Source: CAD feature listing. Evaluate the final solid. Frame: model axes, mm. Face numbers are marked on the shaded views. A direction names the side the tool comes from. Give positions to 0.01 mm unless a question says otherwise; leave off trailing zeros. Write each loop counter-clockwise with the first axis right and the second up, starting at its lowest first coordinate (ties: lowest second). Pieces come first, ordered by that corner, then holes. Notation, with made-up numbers: (-22.5, 13.25) -> (8.5, 13.25) arc R12 ccw to (8.5, 18.25) -> close; hole circle Ø1 at (4, 63). An arc over 180 degrees is marked (long way). Use a Markdown table: item, result. Add a question column.
```python
from build123d import *

# Parameters (mm, degrees)
SFAZOWANIE1_SIZE           = 1
SFAZOWANIE2_SIZE           = 0.5
WYTNIJ_WYCI_GNI_CIE1_START = -25
WYTNIJ_WYCI_GNI_CIE1_DEPTH = 25


with BuildPart() as part:
    # Szkic1 → Obrót1 (revolve)
    with BuildSketch(Plane.XY, mode=Mode.PRIVATE) as obr_t1_sk:
        Polygon((0, 0), (0, 5), (0.6, 5), (0.6, 4.6), (1.7, 4.6), (1.7, 5), (10.7, 5), (10.7, 5.5), (22.7, 5.5), (22.7, 7.5), (47.7, 7.5), (47.7, 10.2), (67.7, 10.2), (67.7, 9.5), (101.7, 9.5), (101.7, 10.2), (121.7, 10.2), (121.7, 12.25), (124.7, 12.25), (124.7, 5), (133.7, 5), (133.7, 4.6), (134.8, 4.6), (134.8, 5), (135.4, 5), (135.4, 0), align=None)
    revolve(obr_t1_sk.sketch.rotate(Axis((-10.674656103, 0, 0), (1, 0, 0)), 90), axis=Axis((-10.674656103, 0, 0), (1, 0, 0)))

    # Sfazowanie1
    # the kernel refuses this chamfer: 1 mm, written as the material it takes off along each edge
    with BuildSketch(Plane(origin=(101.7, 0, 0), x_dir=(0, 0, 1), z_dir=(0, 1, 0))) as sfazowanie1_piece_1_section:
        Polygon((10.2 - SFAZOWANIE1_SIZE, 0), (10.2, SFAZOWANIE1_SIZE), (10.2, 0), align=None)
    sfazowanie1_piece_1 = revolve(axis=Axis((101.7, 0, 0), (1, 0, 0)), mode=Mode.PRIVATE)
    sfazowanie1_piece_1 = sfazowanie1_piece_1 - Plane(origin=(102.341981052, 0, 0), x_dir=(0, 0, 1), z_dir=(1, 0, 0)) * Cylinder(9.5, 41, mode=Mode.PRIVATE)
    add(sfazowanie1_piece_1, mode=Mode.SUBTRACT)
    with BuildSketch(Plane(origin=(67.7, 0, 0), x_dir=(0, 0, 1), z_dir=(0, 1, 0))) as sfazowanie1_piece_2_section:
        Polygon((10.2, -SFAZOWANIE1_SIZE), (10.2 - SFAZOWANIE1_SIZE, 0), (10.2, 0), align=None)
    sfazowanie1_piece_2 = revolve(axis=Axis((67.7, 0, 0), (1, 0, 0)), mode=Mode.PRIVATE)
    sfazowanie1_piece_2 = sfazowanie1_piece_2 - Plane(origin=(67.058018948, 0, 0), x_dir=(0, 0, 1), z_dir=(1, 0, 0)) * Cylinder(9.5, 41, mode=Mode.PRIVATE)
    add(sfazowanie1_piece_2, mode=Mode.SUBTRACT)
    with BuildSketch(Plane(origin=(124.7, 0, 0), x_dir=(0, 0, 1), z_dir=(0, 1, 0))) as sfazowanie1_piece_3:
        Polygon((12.25, -SFAZOWANIE1_SIZE), (12.25 - SFAZOWANIE1_SIZE, 0), (12.25, 0), align=None)
    revolve(axis=Axis((124.7, 0, 0), (1, 0, 0)), mode=Mode.SUBTRACT)
    with BuildSketch(Plane(origin=(47.7, 0, 0), x_dir=(0, 0, 1), z_dir=(0, 1, 0))) as sfazowanie1_piece_4:
        Polygon((10.2 - SFAZOWANIE1_SIZE, 0), (10.2, SFAZOWANIE1_SIZE), (10.2, 0), align=None)
    revolve(axis=Axis((47.7, 0, 0), (1, 0, 0)), mode=Mode.SUBTRACT)

    # Sfazowanie2
    sfazowanie2_edges = [part.edges().sort_by_distance(p)[0] for p in [
        (135.4, 0, -5),
        (0, 0, -5),
    ]]
    chamfer(sfazowanie2_edges, length=SFAZOWANIE2_SIZE)

    # Szkic2 → Wytnij-wyciągnięcie1 (cut)
    with BuildSketch(Plane.ZY.offset(-22.7).offset(WYTNIJ_WYCI_GNI_CIE1_START)):
        with BuildLine():
            Line((4.5, -6), (-4.5, -6))
            ThreePointArc((-4.5, -6), (0, -7.5), (4.5, -6))
        make_face()
    extrude(amount=WYTNIJ_WYCI_GNI_CIE1_DEPTH, mode=Mode.SUBTRACT)


solid = part.part
```
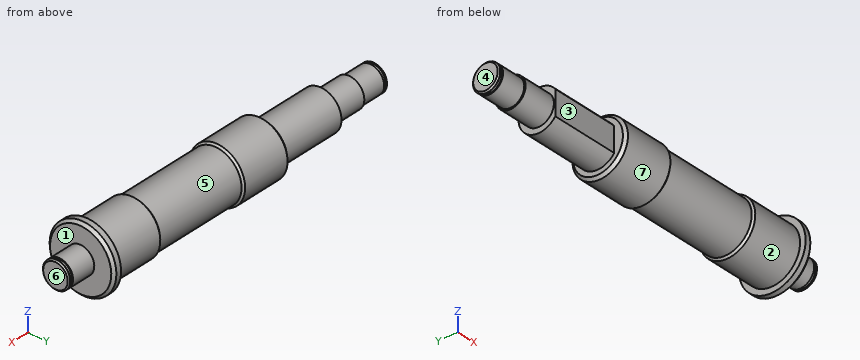
(1) Mould query, pull axis X, two halves, no side actions, for the marked faces 4, 5, 6 and 7. Classes: +X half, -X half, draft (parallel to the pull), parting line (faces both ways), or undercut.
(2) Cut plane B-B on x = 43. Return the cut outline in (y, z), then the cut area to 3 significant figures.
(3) Cut plane A-A on x = 63.5. Return the cut outline in (y, z).
(4) Material intervals for L1, parallel to X at y = -3.75, z = -3; L2, parallel to X at y = 10.5, z = -0.75; L3, parallel to Z at x = 116, y = -0.75, sorted ascending.
(5) Access query for the marked faces 1, 2 and 3. Directions: +Z, -Z, +X, -X, +Y, -Y. A direction counts if a zero-diameter tool reaches every point of the face in a straight line with its end or side. Return the directions, or none.
(6) First-contact query: pin 1 Ø1 at (x, y) = (91, 0.5) entering from -Z; pin 2 Ø5 at (y, z) = (8, 4.5) entering from +X; pin 3 Ø5 at (y, z) = (9, -2.5) entering from -X. Flat tips, straight axial feed; report the tip coordinate or a pass-through.
Output:
| question | item | result |
|---|---|---|
| 1 | face 4 | -X half |
| 1 | face 5 | undercut |
| 1 | face 6 | +X half |
| 1 | face 7 | draft |
| 2 | outline | (-6, -4.5) arc R7.5 ccw (long way) to (-6, 4.5) -> close |
| 2 | area | 168 mm^2 |
| 3 | outline | circle Ø20.4 at (0, 0) |
| 4 | L1 | 0.3 to 0.6, 1.7 to 133.7, 134.8 to 135.1 |
| 4 | L2 | 121.7 to 124.7 |
| 4 | L3 | -10.17 to 10.17 |
| 5 | face 1 | +X |
| 5 | face 2 | -X |
| 5 | face 3 | +Z, -Z, -X, -Y |
| 6 | pin 1 | z = -9.5 |
| 6 | pin 2 | x = 124.7 |
| 6 | pin 3 | x = 22.7 |
